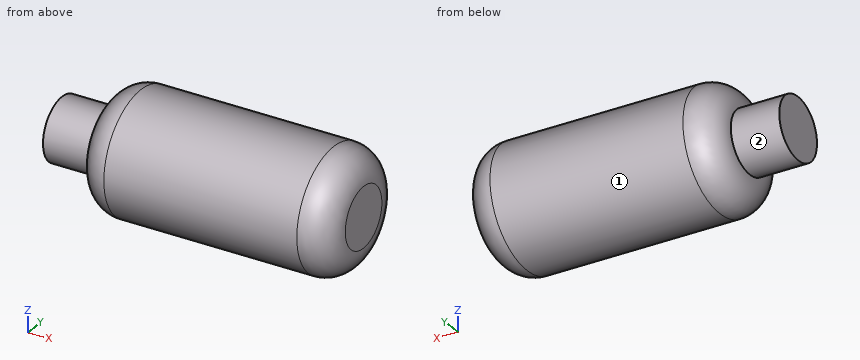
from build123d import *

# Parameters (mm, degrees)
F2_R = 6.35


# Not quite as in the source:
# - a fillet or chamfer that OpenCascade refuses, or shapes differently, is made with other operations: its cross-section is extruded or revolved along the edge and cut away or added


with BuildPart() as f1:
    # F0 (on Front) → F1 (revolve)
    with BuildSketch(Plane.XZ):
        Polygon((-63.5, 0), (0, 0), (0, 12.7), (-53.3020635424, 12.7), (-53.3020635424, 6.5387478179), (-63.5, 6.5387478179), align=None)
    revolve(axis=Axis((-31.75, 0, 0), (-1, 0, 0)))

    # F2
    f2_edges = [f1.edges().sort_by_distance(p)[0] for p in [
        (0, 0, -12.7),
    ]]
    fillet(f2_edges, radius=F2_R)

    # F3: fillet of radius 6.35 on 1 edges, made by hand

    # F3_s1 → F3_t2 (revolve, cut)
    with BuildSketch(Plane.XZ):
        with BuildLine():
            ThreePointArc((-46.9548693385, 12.7), (-51.3777615685, 10.9063718375), (-53.3020635424, 6.5387478179))
            Line((-53.3020635424, 6.5387478179), (-53.3020635424, 12.7))
            Line((-53.3020635424, 12.7), (-46.9548693385, 12.7))
        make_face()
    revolve(axis=Axis((-53.3020635424, 0, 0), (-1, 0, 0)), mode=Mode.SUBTRACT)


solid = f1.part
Model file for the job. Use its own axes, mm. Face numbers are marked on the shaded views. A direction names the side the tool comes from. Give positions to 0.01 mm unless a question says otherwise; leave off trailing zeros. Order: outer loops, then holes, each group sorted by start corner. A loop starts at its lowest first (then second) coordinate and runs counter-clockwise, first axis right, second up. Notation, with made-up numbers: M -28,-0.5 L -18,-0.5 A10 cw -18,3.5 Z; hole C 56,-30 d2. An arc over 180 degrees is marked long. Write item = value, one per line.
Q1. Flat gauge pins, fed straight in: pin 1 (1 mm diameter, centred on x = -38, y = 4.5, fed in from +Z); pin 2 (12 mm diameter, centred on x = -43, z = 7, fed in from -Y); pin 3 (4 mm diameter, centred on y = 6, z = -6.5, fed in from +X). Where does each tip first touch, or does it go through?
Derived:
pin_1 = 12.05
pin_2 = -12.66
pin_3 = -0.02
Q2. Tool access for the marked faces 1 and 2: list every direction of +Z, -Z, +X, -X, +Y, -Y with a clear straight run to the whole face (end or side of a thin tool).
Derived:
face_1 = +X, -X
face_2 = -X
Q3. Drill centre lines: line 1 (Z direction, x = -25.5, y = -0.5); line 2 (Y direction, x = -7.5, z = 0); line 3 (Z direction, x = -22, y = 9). Where is each one in solid material? Low to high. Write a range as [from, to].
Derived:
line_1 = [-12.69, 12.69]
line_2 = [-12.7, 12.7]
line_3 = [-8.96, 8.96]
Q4. Cut at A-A, the plane x = -17. List the corners of the cut face in (y, z).
Derived:
outline = C 0,0 d25.4
